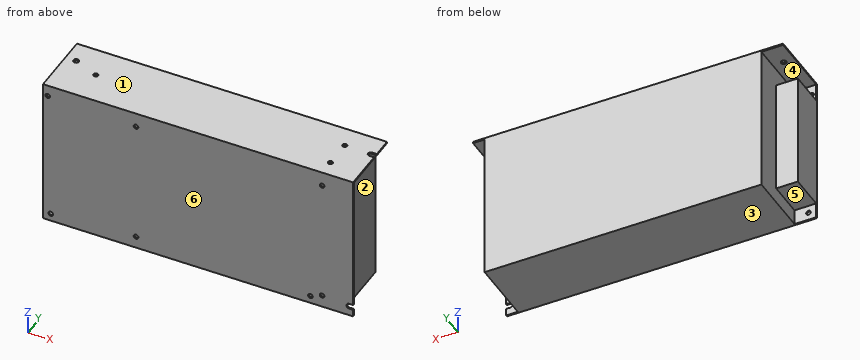
```python
from build123d import *

# Parameters (mm, degrees)
SKETCH1_R           = 1.5
BOSS_EXTRUDE1_DEPTH = 42.5
SKETCH2_W           = 7.5
SKETCH2_H           = 96.5
SKETCH2_W_2         = 14
CUT_EXTRUDE1_DEPTH  = 41.5
CUT_EXTRUDE2_REACH  = 99.5
SKETCH3_R           = 1.75
SKETCH4_W           = 14
SKETCH4_H           = 75
BOSS_EXTRUDE2_DEPTH = 23
SKETCH5_R           = 1.5
CUT_EXTRUDE3_DEPTH  = 1
SKETCH6_R           = 1.5
CUT_EXTRUDE4_DEPTH  = 1


with BuildPart() as part:
    # Sketch1 → Boss-Extrude1 (new body)
    with BuildSketch(Plane(origin=(0, 0, 0), x_dir=(1, 0, 0), z_dir=(0, 1, 0))):
        with BuildLine():
            Line((197.5, 92.75), (200, 92.75))
            Line((200, 92.75), (200, 97.5))
            Line((200, 97.5), (0, 97.5))
            Line((0, 97.5), (0, 0))
            Line((0, 0), (200, 0))
            Line((200, 0), (200, 89.25))
            Line((200, 89.25), (197.5, 89.25))
            ThreePointArc((197.5, 89.25), (195.75, 91), (197.5, 92.75))
        make_face()
        with Locations((3, 7.5)):
            Circle(SKETCH1_R, mode=Mode.SUBTRACT)
    extrude(amount=BOSS_EXTRUDE1_DEPTH)

    # Sketch2 → Cut-Extrude1 (cut)
    with BuildSketch(Plane(origin=(0, 42.5, 0), x_dir=(1, 0, 0), z_dir=(0, 1, 0))):
        with Locations((196.25, 49.25)):
            Rectangle(SKETCH2_W, SKETCH2_H)
        with Locations((7, 49.25)):
            Rectangle(SKETCH2_W_2, SKETCH2_H)
    extrude(amount=-CUT_EXTRUDE1_DEPTH, mode=Mode.SUBTRACT)

    # Sketch3 → Cut-Extrude2 (cut, up to next)
    with BuildSketch(Plane.XY, mode=Mode.PRIVATE) as cut_extrude2_sk1:
        with Locations((7, 28)):
            Circle(SKETCH3_R)
    cut_extrude2_tool1 = extrude(cut_extrude2_sk1.sketch, amount=-CUT_EXTRUDE2_REACH, mode=Mode.PRIVATE) & part.part
    add(cut_extrude2_tool1.solids().sort_by_distance((7, 28, 0))[0], mode=Mode.SUBTRACT)
    # Sketch3 → Cut-Extrude2 (cut, up to next)
    with BuildSketch(Plane.XY, mode=Mode.PRIVATE) as cut_extrude2_sk2:
        with BuildLine():
            Line((197, 29.75), (200, 29.75))
            Line((200, 29.75), (200, 26.25))
            Line((200, 26.25), (197, 26.25))
            ThreePointArc((197, 26.25), (195.25, 28), (197, 29.75))
        make_face()
    cut_extrude2_tool2 = extrude(cut_extrude2_sk2.sketch, amount=-CUT_EXTRUDE2_REACH, mode=Mode.PRIVATE) & part.part
    add(cut_extrude2_tool2.solids().sort_by_distance((197.795339, 28, 0))[0], mode=Mode.SUBTRACT)

    # Sketch4 → Boss-Extrude2 (add)
    with BuildSketch(Plane(origin=(0, 1, 0), x_dir=(1, 0, 0), z_dir=(0, 1, 0))):
        with Locations((7, 50)):
            Rectangle(SKETCH4_W, SKETCH4_H)
    extrude(amount=BOSS_EXTRUDE2_DEPTH)

    # Sketch5 → Cut-Extrude3 (cut)
    with BuildSketch(Plane.XY):
        with Locations((23, 21.5)):
            Circle(SKETCH5_R)
        with Locations((180, 10.5)):
            Circle(SKETCH5_R)
        with Locations((180, 28.5)):
            Circle(SKETCH5_R)
    extrude(amount=-CUT_EXTRUDE3_DEPTH, mode=Mode.SUBTRACT)

    # Sketch6 → Cut-Extrude4 (cut)
    with BuildSketch(Plane.XZ):
        with Locations((5, -92.5)):
            Circle(SKETCH6_R)
        with Locations((60, -9.5)):
            Circle(SKETCH6_R)
        with Locations((60, -89.5)):
            Circle(SKETCH6_R)
        with Locations((180, -89.5)):
            Circle(SKETCH6_R)
        with Locations((180, -9.5)):
            Circle(SKETCH6_R)
        with Locations((172.5, -92.5)):
            Circle(SKETCH6_R)
    extrude(amount=-CUT_EXTRUDE4_DEPTH, mode=Mode.SUBTRACT)


solid = part.part
```
Geometry check sheet. Reference: the model listing, model coordinates, mm. Face numbers are marked on the shaded views. A direction names the side the tool comes from. Coordinates: 2 decimals unless noted, no trailing zeros. Write each loop counter-clockwise with the first axis right and the second up, starting at its lowest first coordinate (ties: lowest second). Pieces come first, ordered by that corner, then holes. Notation, with made-up numbers: M 0.5,34 L 49.5,34 A23 ccw 49.5,71 Z; hole C 60.5,-29.5 d7. An arc over 180 degrees is marked long. Use one line per item in the form item = value. Start each with the question number.
1) Section check B-B on z = -31.5. Enter the section's corners in (x, y), and give its area (3 significant figures).
2) Release check for a two-part mould opening along Z. For the marked faces 1, 2, 3 and 4 record: pulls with the +Z half, pulls with the -Z half, needs draft (parallel to the pull), parting line crosses it, or undercut.
3) Go/stop test with flat-tipped pins: pin 1 Ø0.9 at (x, z) = (179.5, -10) entering from -Y; pin 2 Ø12.5 at (y, z) = (14.5, -40.5) entering from +X; pin 3 Ø4 at (x, y) = (7, 28) entering from -Z. Record where each tip stops, or that it passes through.
4) Set-up check for the marked faces 5 and 6: record each of +Z, -Z, +X, -X, +Y, -Y from which the full face is reachable in a straight line by a thin tool's end or side.
5) Thickness scan on probe 1 along Z at (x, y) = (60, 0.45); probe 2 along Y at (x, z) = (180, -0.5); probe 3 along X at (y, z) = (0.4, -92.5). Record the ranges inside material, lowest first. Write a range as from..to.
6) Section check A-A on y = 36.5. Enter the section's corners in (x, z).
Responses:
q1.outline = M 0,0 L 200,0 L 200,1 L 192.5,1 L 192.5,42.5 L 14,42.5 L 14,24 L 0,24 Z
q1.area = 7,930 mm2
q2.face_1 = pulls with the +Z half
q2.face_2 = needs draft
q2.face_3 = pulls with the -Z half
q2.face_4 = undercut
q3.pin_1 = 1
q3.pin_2 = 192.5
q3.pin_3 = -1
q4.face_5 = -Z, -X, +Y
q4.face_6 = +Z, -Z, +X, -X, -Y
q5.probe_1 = -97.5..-91, -88..-11, -8..0
q5.probe_2 = 0..9, 12..27, 30..42.5
q5.probe_3 = 0..3.5, 6.5..171, 174..196.6
q6.outline = M 0,-1 L 14,-1 L 14,-97.5 L 192.5,-97.5 L 192.5,-1 L 200,-1 L 200,0 L 0,0 Z
